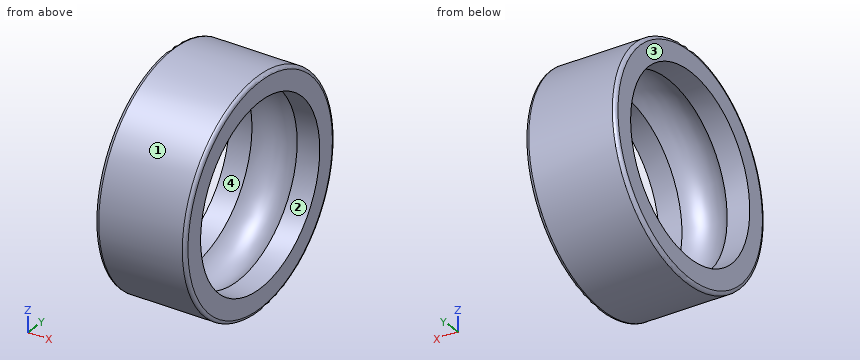
from build123d import *

# Parameters (mm, degrees)
CONG_1_R = 0.15


with BuildPart() as part:
    # Esquisse1 → Base-Révolution (revolve)
    with BuildSketch(Plane.XY):
        with BuildLine():
            Line((0, 4), (1, 4))
            ThreePointArc((1, 4), (2, 4.5), (3, 4))
            Line((3, 4), (4, 4))
            Line((4, 4), (4, 5))
            Line((4, 5), (0, 5))
            Line((0, 5), (0, 4))
        make_face()
    revolve(axis=Axis((0, 0, 0), (1, 0, 0)))

    # Congé1
    cong_1_edges = [part.edges().sort_by_distance(p)[0] for p in [
        (4, -5, 0),
        (0, -5, 0),
    ]]
    fillet(cong_1_edges, radius=CONG_1_R)


solid = part.part
Geometry check sheet. Reference: the model listing, model coordinates, mm. Face numbers are marked on the shaded views. Round coordinates to 2 decimals unless told otherwise and drop trailing zeros. Order: outer loops, then holes, each group sorted by start corner. A loop starts at its lowest first (then second) coordinate and runs counter-clockwise, first axis right, second up. Notation, with made-up numbers: M 13.5,3 L 24.5,3 A20 cw 24.5,22 Z; hole C 41,11.5 d11. An arc over 180 degrees is marked long. Answer in a Markdown table with one row per item. Add a question column.
Item 1: Sectioned sample at A-A, the plane z = 0. Enter the section's corners in (x, y), plus the area to 3 significant figures.
Item 2: Depth check by flat-ended pin: pin 1 Ø2 at (x, z) = (1.5, -3) entering from +Y; pin 2 Ø1.5 at (x, z) = (3.5, -1) entering from +Y; pin 3 Ø5 at (y, z) = (0, 0) entering from -X; pin 4 Ø1.5 at (x, y) = (2.5, 1.5) entering from -Z. Enter the tip coordinate at first touch or a pass-through.
Item 3: Material ranges on L1, parallel to Z at x = 3.75, y = 0; L2, parallel to Z at x = 2.35, y = 1; L3, parallel to Y at x = 1.3, z = 3.25, recorded low to high. Write a range as [from, to].
Item 4: Draft check along Z on the marked faces 1, 2, 3 and 4. Enter one of: released by +Z, released by -Z, zero draft, split by the parting line, or undercut.
Item 5: Sectioned sample at C-C, the plane x = 2.4. Enter the section's corners in (y, z).
Filled in:
| question | item | result |
|---|---|---|
| 1 | outline | M 0,-4.85 A0.15 ccw 0.15,-5 L 3.85,-5 A0.15 ccw 4,-4.85 L 4,-4 L 3,-4 A1.25 cw 1,-4 L 0,-4 Z; M 0,4 L 1,4 A1.25 cw 3,4 L 4,4 L 4,4.85 A0.15 ccw 3.85,5 L 0.15,5 A0.15 ccw 0,4.85 Z |
| 1 | area | 6.58 mm² |
| 2 | pin 1 | stops at y = 4.58 |
| 2 | pin 2 | stops at y = 4.99 |
| 2 | pin 3 | passes through |
| 2 | pin 4 | stops at z = -4.94 |
| 3 | L1 | z = [-5, -4], [4, 5] |
| 3 | L2 | z = [-4.9, -4.34], [4.34, 4.9] |
| 3 | L3 | y = [-3.8, -2.79], [2.79, 3.8] |
| 4 | face 1 | split by the parting line |
| 4 | face 2 | undercut |
| 4 | face 3 | zero draft |
| 4 | face 4 | undercut |
| 5 | outline | C 0,0 d10; hole C 0,0 d8.87 |
